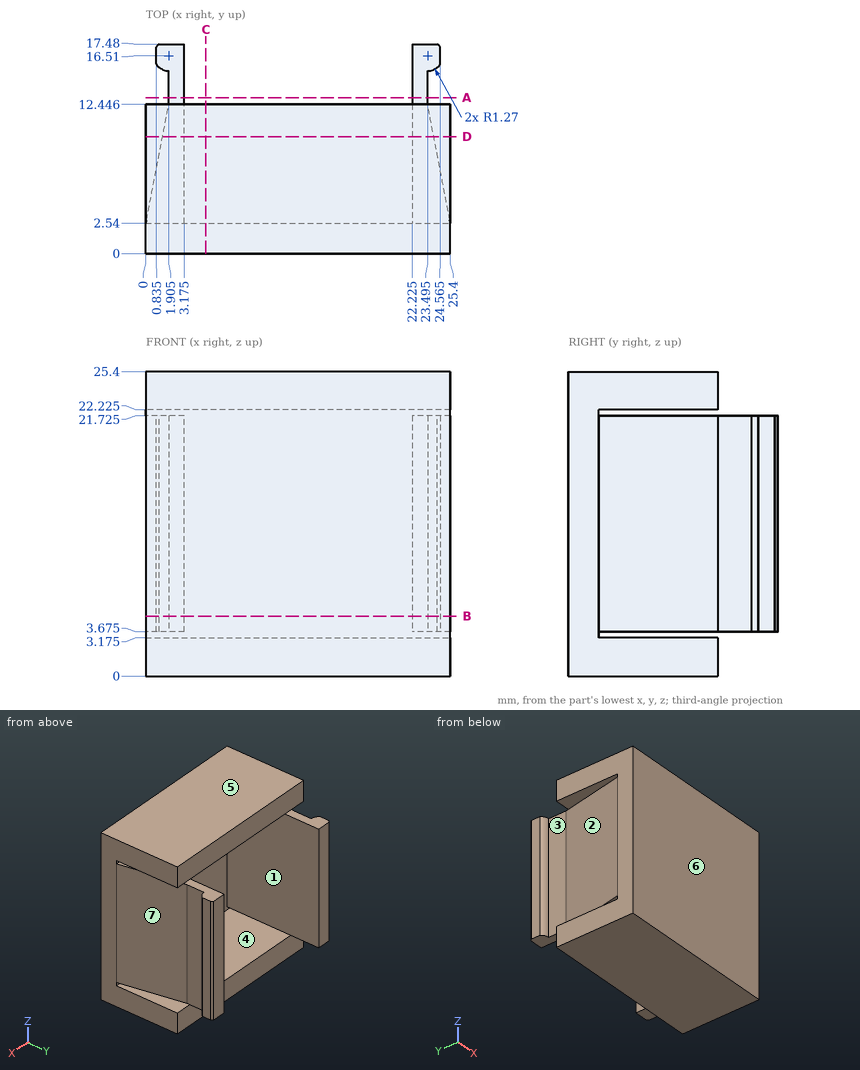
Can you work these out from the drawing? Everything is in mm from the part's minimum corner. A direction names the side the tool comes from. Coordinates: 2 decimals unless noted, no trailing zeros. Loops run counter-clockwise (first coordinate to the right, second up) from the corner with the lowest first, then second, coordinate; pieces in that order, holes last. Notation, with made-up numbers: (38.5, 62.5) - (72.5, 62.5) arc R13 ccw to (72.5, 86.5) - close; hole circle Ø9 at (-16, -14). An arc over 180 degrees is marked (long way). Put each result on its own line as item: value. Start each with the question number.
Item 1: Suppose I cut it at B-B (z = 5). Please give me the cut outline in (x, y) (3 decimals), and give its area (3 significant figures).
Item 2: Which directions (+Z, -Z, +X, -X, +Y, -Y) give clear straight access to the entire face, cutting with the end or side of a thin tool? Please do the marked faces 1, 2, 3 and 4.
Item 3: Suppose I cut it at D-D (y = 9.75). Please give me the cut outline in (x, z) (3 decimals), and give its area (3 significant figures).
Item 4: If we mould it in two halves opening along Z, with no side actions, what happens to the marked faces 5, 6 and 7? For each: +Z half, -Z half, draft (parallel to the pull), parting line (faces both ways), or undercut.
Item 5: If I drill on line 1 along Z through (x, y) = (1.5, 9.75) (3 decimals); line 2 along X through (y, z) = (14.5, 17) (3 decimals); line 3 along Z through (x, y) = (9.25, 5.5) (3 decimals), over which ranges is the centre line in solid material (lowest first)?
Item 6: Suppose I cut it at C-C (x = 5). Please give me the cut outline in (y, z) (3 decimals), and give its area (3 significant figures).
Item 7: Suppose I cut it at A-A (y = 13). Please give me the cut outline in (x, z) (3 decimals).
Item 8: For pin 1 (2.5 mm diameter, centred on x = 7.5, z = 24.5, fed in from +Y); pin 2 (1.1 mm diameter, centred on y = 16, z = 10.5, fed in from +X) (3 decimals); pin 3 (1 mm diameter, centred on x = 21, z = 4, fed in from +Y); pin 4 (3 mm diameter, centred on x = 5, y = 14.5, fed in from +Z), each with a flat end and sliding along its axis, tell me the tip position at first contact or that it passes through.
Here are the results:
1. outline: (0, 0) - (25.4, 0) - (25.4, 2.54) - (23.495, 12.446) - (23.495, 15.24) arc R1.27 ccw to (24.565, 15.826) - (24.565, 17.194) arc R1.27 ccw to (24.315, 17.48) - (22.225, 17.48) - (22.225, 2.54) - (3.175, 2.54) - (3.175, 17.48) - (1.085, 17.48) arc R1.27 ccw to (0.835, 17.194) - (0.835, 15.826) arc R1.27 ccw to (1.905, 15.24) - (1.905, 12.446) - (0, 2.54) - close
1. area: 126 mm²
2. face 1: +Y
2. face 2: -X
2. face 3: +Z, -Z, -X
2. face 4: +X, -X, +Y
3. outline: (0, 0) - (25.4, 0) - (25.4, 3.175) - (0, 3.175) - close; (0, 22.225) - (25.4, 22.225) - (25.4, 25.4) - (0, 25.4) - close; (1.387, 3.675) - (3.175, 3.675) - (3.175, 21.725) - (1.387, 21.725) - close; (22.225, 3.675) - (24.013, 3.675) - (24.013, 21.725) - (22.225, 21.725) - close
3. area: 226 mm²
4. face 5: +Z half
4. face 6: draft
4. face 7: undercut
5. line 1: 0 to 3.175, 3.675 to 21.725, 22.225 to 25.4
5. line 2: 1.905 to 3.175, 22.225 to 23.495
5. line 3: 0 to 3.175, 22.225 to 25.4
6. outline: (0, 0) - (12.446, 0) - (12.446, 3.175) - (2.54, 3.175) - (2.54, 22.225) - (12.446, 22.225) - (12.446, 25.4) - (0, 25.4) - close
6. area: 127 mm²
7. outline: (1.905, 3.675) - (3.175, 3.675) - (3.175, 21.725) - (1.905, 21.725) - close; (22.225, 3.675) - (23.495, 3.675) - (23.495, 21.725) - (22.225, 21.725) - close
8. pin 1: y = 12.45
8. pin 2: x = 24.565
8. pin 3: y = 2.54
8. pin 4: through
